Autodesk Inventor part; units mm, degrees
ref_plane "YZ Plane" through (0, 0, 0) normal (1, 0, 0) x (0, 1, 0)
ref_plane "XZ Plane" through (0, 0, 0) normal (0, 1, 0) x (-1, 0, 0)
ref_plane "XY Plane" through (0, 0, 0) normal (0, 0, 1) x (1, 0, 0)
sketch "Sketch1" plane through (0, 0, 0) normal (0, 1, 0) x (-1, 0, 0)
  line L0 (2.3057, -4.7625) -> (-8.7313, -4.7625)
  line L1 (-7.1437, 4.7625) -> (7.1438, 4.7625)
  line L2 (8.7313, -4.7625) -> (-8.7313, 4.7625) construction
  line L3 (-8.7313, -4.7625) -> (8.7313, 4.7625) construction
  arc A0 (8.7313, 3.175) -> (7.1438, 4.7625) centre (7.1438, 3.175) ccw
  arc A1 (-7.1437, 4.7625) -> (-8.7313, 3.175) centre (-7.1437, 3.175) ccw
  line L4 (0, -4.7625) -> (-1.5875, -4.7625)
  line L5 (0, -4.7625) -> (1.5875, -4.7625)
  arc A2 (1.5875, -4.7625) -> (8.7313, 3.175) centre (1.9466, 2.0978) ccw
  line L6 (0, -11.8883) -> (0, 12.0323) construction
  arc A3 (-8.7313, 3.175) -> (-1.5875, -4.7625) centre (-1.9466, 2.0978) ccw
  point P0 (0, 0)
  point P1 (-2.3057, -4.7625)
  dimension "d0" = 17.4625
  dimension "d1" = 9.525
  dimension "d2" = 1.5875
  dimension "d3" = 1.5875
  dimension "d4" = 1.5875
  dimension "d5" = 1.5875
extrude "Extrusion1" add sketch "Sketch1" along normal blind 19.05 contours L0 A3 A1 L1 A0 A2
sketch "Sketch2" plane through (0, 19.05, 0) normal (0, 1, 0) x (1, 0, 0)
  line L0 (-7.1438, -4.7625) -> (7.1437, -4.7625)
  line L1 (8.8162, 2.8402) -> (8.8162, -4.7625) construction
  arc A0 (8.7313, -3.175) -> (2.3057, 4.7625) centre (1.9466, -2.0978) ccw construction
  line L2 (4.0537, -4.7625) -> (4.6092, -3.5183)
  line L3 (5.0753, -3.3835) -> (7.1437, -4.7625)
  line L4 (4.0537, -4.7625) -> (7.1437, -4.7625)
  arc A1 (5.0753, -3.3835) -> (4.6092, -3.5183) centre (4.8992, -3.6477) ccw
  line L5 (4.0537, -4.7625) -> (7.1437, -4.7625)
  line L6 (4.0537, -4.7625) -> (7.1437, -4.7625)
  line L7 (2.3057, 4.7625) -> (-2.3057, 4.7625) construction
  line L8 (0, 4.7625) -> (0, -4.7625) construction
  line L9 (-4.0537, -4.7625) -> (-4.6092, -3.5183)
  line L10 (-5.0753, -3.3835) -> (-7.1438, -4.7625)
  line L11 (-4.0537, -4.7625) -> (-7.1438, -4.7625)
  arc A2 (-4.6092, -3.5183) -> (-5.0753, -3.3835) centre (-4.8992, -3.6477) ccw
  line L12 (-4.0537, -4.7625) -> (-7.1438, -4.7625)
  line L13 (-4.0537, -4.7625) -> (-7.1438, -4.7625)
  point P0 (0, 0)
  dimension "d8" = 4.7625
  dimension "d9" = 0.3175
extrude "Extrusion2" cut sketch "Sketch2" against normal blind 19.05
sketch "Sketch3" plane through (-4.0537, 0, 4.7625) normal (0, 0, 1) x (1, 0, 0)
  circle A0 centre (4.0537, 12.7) radius 1.5875
  line L0 (0, 0) -> (8.1075, 0)
  point P0 (4.0537, 0)
  dimension "d12" = 3.175
  dimension "d13" = 12.7
extrude "Extrusion3" cut sketch "Sketch3" against normal blind 19.05
properties part number "Curved Slider v1.0"
Design review of the part built by this model. Coordinates are the model's own, in mm. A direction names the side the tool comes from. Give positions to 0.01 mm unless a question says otherwise; leave off trailing zeros. Order: outer loops, then holes, each group sorted by start corner. A loop starts at its lowest first (then second) coordinate and runs counter-clockwise, first axis right, second up. Notation, with made-up numbers: (14, 74.25) - (67, 74.25) arc R16 ccw to (67, 101.25) - close; hole circle Ø3 at (-36.5, 48). An arc over 180 degrees is marked (long way). Use a Markdown table: item, result. Add a question column.
(1) Clearance check with flat-ended pins moving along their axes: P1, Ø3, axis at y = 13.5, z = -0.5, coming from the +X side; P2, Ø1.5, axis at y = 11.5, z = 3.5, coming from the -X side; P3, Ø2, axis at y = 10.5, z = -1.5, coming from the +X side. State where each tip first meets the part, or that it passes through.
(2) Add section C-C on z = 3.75. Give the number of separate pieces and of enclosed holes in the cut face, then the cut area to 3 significant figures.
(3) Machinability: for faces 4 (the face through (8.279, 9.392, 4.285)), 5 (the face through (-6, 10, 4)), which of the approach directions +Z, -Z, +X, -X, +Y, -Y give a long, thin tool a straight path to every point of the face, cutting with its end or side? Answer none if there is none.
(4) Add section A-A on x = 0. Give the boundary of the cut face in (y, z), then the cut area to 3 significant figures.
(5) Add section B-B on y = 12.7. Give the boundary of the cut face in (x, z) (1 decimal).
(6) Add section D-D on y = 15.25. Give the boundary of the cut face in (x, z) (1 decimal), then the cut area to 3 significant figures.
(7) Wall thickness on probe 1 along Y at (x, z) = (0, 0.5); probe 2 along X at (y, z) = (3, 3.5); probe 3 along X at (y, z) = (14, 2.25): over which ranges is each line inside the solid? List them lowest first. Write a range as [from, to].
(8) Mouldability with a two-part tool opening along X and no side actions: class faces 1 (the face through (0, 9, 4.762)), 2 (the face through (6, 10, 4)), 3 (the face through (-8.254, 9.392, 4.31)) as +X half, -X half, draft (parallel to the pull), parting line (faces both ways), or undercut.
Report:
| question | item | result |
|---|---|---|
| 1 | P1 | stops at x = 8.73 |
| 1 | P2 | stops at x = -8.79 |
| 1 | P3 | stops at x = 8.31 |
| 2 | separate pieces | 3 |
| 2 | enclosed holes | 1 |
| 2 | area | 278 mm² |
| 3 | face 4 | +Z, +X, +Y, -Y |
| 3 | face 5 | +Z, +Y, -Y |
| 4 | outline | (0, -4.76) - (11.11, -4.76) - (11.11, 4.76) - (0, 4.76) - close; (14.29, -4.76) - (19.05, -4.76) - (19.05, 4.76) - (14.29, 4.76) - close |
| 4 | area | 151 mm² |
| 5 | outline | (-8.7, 3.2) arc R6.9 ccw to (-2.3, -4.8) - (-1.6, -4.8) - (-1.6, 4.8) - (-4.1, 4.8) - (-4.6, 3.5) arc R0.3 cw to (-5.1, 3.4) - (-7.1, 4.8) arc R1.6 ccw to start; (1.6, -4.8) - (2.3, -4.8) arc R6.9 ccw to (8.7, 3.2) arc R1.6 ccw to (7.1, 4.8) - (5.1, 3.4) arc R0.3 cw to (4.6, 3.5) - (4.1, 4.8) - (1.6, 4.8) - close |
| 6 | outline | (-8.7, 3.2) arc R6.9 ccw to (-2.3, -4.8) - (2.3, -4.8) arc R6.9 ccw to (8.7, 3.2) arc R1.6 ccw to (7.1, 4.8) - (5.1, 3.4) arc R0.3 cw to (4.6, 3.5) - (4.1, 4.8) - (-4.1, 4.8) - (-4.6, 3.5) arc R0.3 cw to (-5.1, 3.4) - (-7.1, 4.8) arc R1.6 ccw to start |
| 6 | area | 142 mm² |
| 7 | probe 1 | y = [0, 11.11], [14.29, 19.05] |
| 7 | probe 2 | x = [-8.7, -5.25], [-4.62, 4.62], [5.25, 8.7] |
| 7 | probe 3 | x = [-8.81, -0.91], [0.91, 8.81] |
| 8 | face 1 | draft |
| 8 | face 2 | undercut |
| 8 | face 3 | -X half |
